Answer from the drawing. Dimensions are ordinates in mm from the lowest x, y and z of the part. A direction names the side the tool comes from. Coordinates: 2 decimals unless noted, no trailing zeros. Write each loop counter-clockwise with the first axis right and the second up, starting at its lowest first coordinate (ties: lowest second). Pieces come first, ordered by that corner, then holes. Notation, with made-up numbers: (55.25, 86.25) -> (82.25, 86.25) arc R24 ccw to (82.25, 124.25) -> close; hole circle Ø11 at (-39, -11.5). An arc over 180 degrees is marked (long way). One line per item, written item: value. Start each with the question number.
1. Find section C-C, the plane z = 126. Write down the section's boundary in (x, y), and give its area (3 significant figures).
2. Find section B-B, the plane x = 180. Write down the section's boundary in (y, z), and give its area (3 significant figures).
3. For a pull along X with two mould halves and no side action, classify the marked faces 1, 2, 3 and 4 as pulls with the +X half, pulls with the -X half, needs draft (parallel to the pull), parting line crosses it, or undercut.
4. Find section A-A, the plane y = 512. Write down the section's boundary in (x, z).
5. Consider line 1 along X through (y, z) = (643.5, 178); line 2 along Y through (x, z) = (285, 243); line 3 along Y through (x, z) = (196, 160). Determine where each line is inside the solid, lowest interval first.
6. Given P1, Ø8, axis at x = 159.5, y = 187.5, coming from the +Z side; P2, Ø2, axis at x = 296, z = 231.5, coming from the +Y side; P3, Ø4, axis at x = 101, z = 130, coming from the -Y side, each flat-ended and moving along its own axis, determine where each tip first touches the part or whether it passes through.
7. For the marked faces 5, 6 and 7, determine the directions among +Z, -Z, +X, -X, +Y, -Y from which every point of the face is accessible in a straight line to the end or side of a thin tool.
8. Find section D-D, the plane y = 308.5. Write down the section's boundary in (x, z), and give its area (3 significant figures).
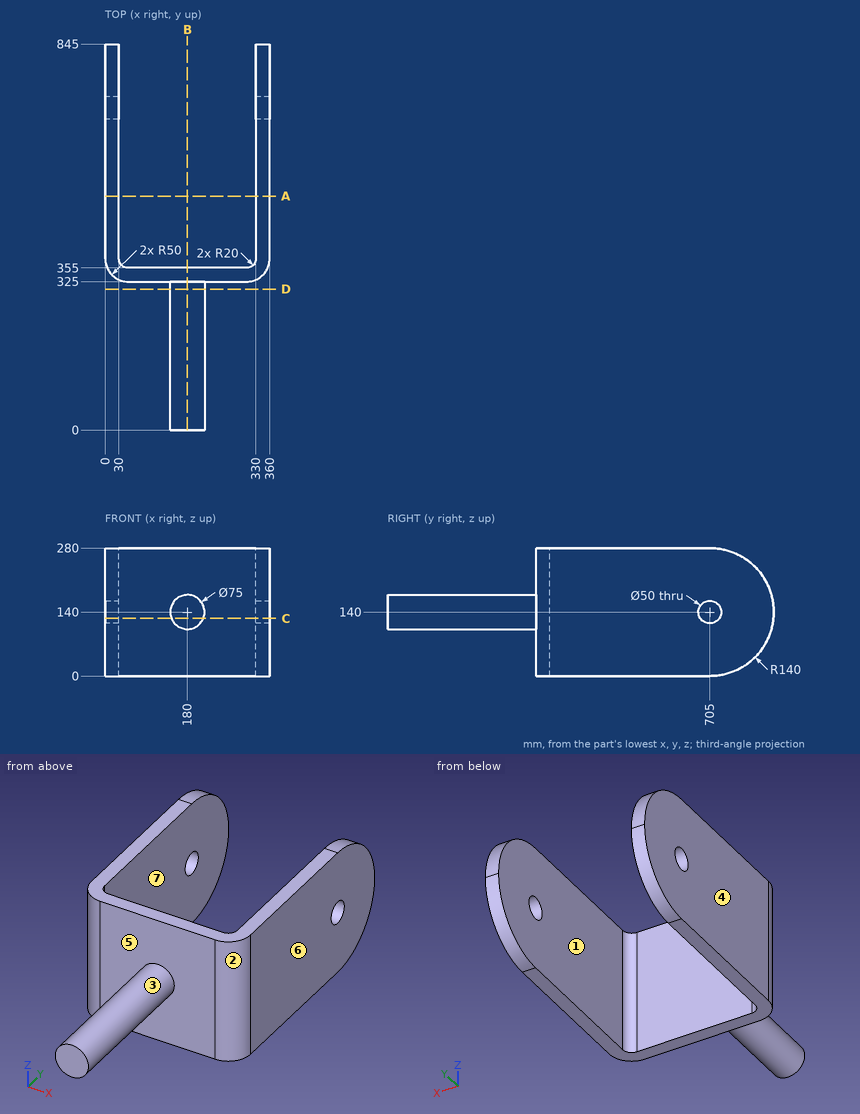
Answer block:
1. outline: (0, 375) arc R50 ccw to (50, 325) -> (145.21, 325) -> (145.21, 0) -> (214.79, 0) -> (214.79, 325) -> (310, 325) arc R50 ccw to (360, 375) -> (360, 684.29) -> (330, 684.29) -> (330, 375) arc R20 cw to (310, 355) -> (50, 355) arc R20 cw to (30, 375) -> (30, 684.29) -> (0, 684.29) -> close; (0, 725.71) -> (30, 725.71) -> (30, 844.3) -> (0, 844.3) -> close; (330, 725.71) -> (360, 725.71) -> (360, 844.3) -> (330, 844.3) -> close
1. area: 59,400 mm2
2. outline: (0, 102.5) -> (325, 102.5) -> (325, 0) -> (355, 0) -> (355, 280) -> (325, 280) -> (325, 177.5) -> (0, 177.5) -> close
2. area: 32,800 mm2
3. face 1: undercut
3. face 2: pulls with the +X half
3. face 3: parting line crosses it
3. face 4: pulls with the -X half
4. outline: (0, 0) -> (30, 0) -> (30, 280) -> (0, 280) -> close; (330, 0) -> (360, 0) -> (360, 280) -> (330, 280) -> close
5. line 1: x = 0 to 30, 330 to 360
5. line 2: y = 325 to 355
5. line 3: y = 0 to 355
6. P1: stops at z = 173.67
6. P2: stops at y = 355
6. P3: stops at y = 325
7. face 5: -Y
7. face 6: +Z, -Z, +X, +Y, -Y
7. face 7: +Z, -Z, +Y
8. outline: circle Ø75 at (180, 140)
8. area: 4,420 mm2
